Read the model definition and answer for the solid it produces. Units are mm, in the model's axes. A direction names the side the tool comes from. Give positions to 0.01 mm unless a question says otherwise; leave off trailing zeros. Order: outer loops, then holes, each group sorted by start corner. A loop starts at its lowest first (then second) coordinate and runs counter-clockwise, first axis right, second up.
Item 1: A cutting plane is placed at C-C (y = -8.5). Write down the section's boundary in (x, z).
Item 2: Which of the six approach directions +Z, -Z, +X, -X, +Y, -Y give full straight-line access (tool end or side, diameter ignored) to faces 1 (the face through (-9.19, -17.68, 3.45)), 2 (the face through (5.75, 6.62, 3.45))?
Item 3: Find the intervals of material crossed by line 1 along Y through (x, z) = (-3.75, 2.5); line 2 along Y through (x, z) = (-4.25, 5.5); line 3 along X through (y, z) = (-10, 3.75), in increasing order.
Item 4: The mould has two halves that part along X. Classify faces 3 (the face through (10.2, 0, 3)), 4 (the face through (5.8, -6.71, 3.45)), 5 (the face through (-9.19, 17.68, 3.45)), 6 (the face through (0, 18.668, 3)): +X half, -X half, draft (parallel to the pull), parting line (faces both ways), or undercut.
Item 5: A cutting plane is placed at B-B (z = 0.5). Write down the section's boundary in (x, y), plus the area to 3 significant figures.
Item 6: Given pin 1 Ø2 at (x, y) = (6, -1) entering from -Z, flat-ended and moving along its own axis, determine where the tip first touches the part or whether it passes through.
Item 7: A cutting plane is placed at D-D (x = 4.25). Write down the section's boundary in (y, z), plus the area to 3 significant figures.
Item 8: A cutting plane is placed at A-A (x = 1.5). Write down the section's boundary in (y, z), plus the area to 3 significant figures.
from build123d import *

# Parameters (mm, degrees)
SKETCH_W     = 20.4
SKETCH_H     = 37.336792
PAD_DEPTH    = 7
CHAMFER_SIZE = 2


with BuildPart() as part:
    # Sketch → Pad (new body)
    with BuildSketch(Plane.XY):
        Rectangle(SKETCH_W, SKETCH_H)
        Polygon((3.85, 16.668396), (-3.85, 16.668396), (-7.7, 10), (-3.85, 3.331604), (3.85, 3.331604), (7.7, 10), align=None, mode=Mode.SUBTRACT)
        Polygon((3.85, -3.331604), (-3.85, -3.331604), (-7.7, -10), (-3.85, -16.668396), (3.85, -16.668396), (7.7, -10), align=None, mode=Mode.SUBTRACT)
    extrude(amount=PAD_DEPTH)

    # Chamfer
    chamfer_edges = [part.edges().sort_by_distance(p)[0] for p in [
        (10.2, 18.668396, 3.5),
        (-10.2, 18.668396, 3.5),
        (10.2, -18.668396, 3.5),
        (-10.2, -18.668396, 3.5),
    ]]
    chamfer(chamfer_edges, length=CHAMFER_SIZE)


solid = part.part
Response values:
1. outline: (-10.2, 0) - (-6.83, 0) - (-6.83, 7) - (-10.2, 7) - close; (6.83, 0) - (10.2, 0) - (10.2, 7) - (6.83, 7) - close
2. face 1: +Z, -Z, -X, -Y
2. face 2: +Z, -Z
3. line 1: y = -18.67 to -16.67, -3.33 to 3.33, 16.67 to 18.67
3. line 2: y = -18.67 to -15.98, -4.02 to 4.02, 15.98 to 18.67
3. line 3: x = -10.2 to -7.7, 7.7 to 10.2
4. face 3: +X half
4. face 4: undercut
4. face 5: -X half
4. face 6: draft
5. outline: (-10.2, -16.67) - (-8.2, -18.67) - (8.2, -18.67) - (10.2, -16.67) - (10.2, 16.67) - (8.2, 18.67) - (-8.2, 18.67) - (-10.2, 16.67) - close; hole (-7.7, -10) - (-3.85, -16.67) - (3.85, -16.67) - (7.7, -10) - (3.85, -3.33) - (-3.85, -3.33) - close; hole (-7.7, 10) - (-3.85, 3.33) - (3.85, 3.33) - (7.7, 10) - (3.85, 16.67) - (-3.85, 16.67) - close
5. area: 446 mm2
6. pin 1: stops at z = 0
7. outline: (-18.67, 0) - (-15.98, 0) - (-15.98, 7) - (-18.67, 7) - close; (-4.02, 0) - (4.02, 0) - (4.02, 7) - (-4.02, 7) - close; (15.98, 0) - (18.67, 0) - (18.67, 7) - (15.98, 7) - close
7. area: 94.0 mm2
8. outline: (-18.67, 0) - (-16.67, 0) - (-16.67, 7) - (-18.67, 7) - close; (-3.33, 0) - (3.33, 0) - (3.33, 7) - (-3.33, 7) - close; (16.67, 0) - (18.67, 0) - (18.67, 7) - (16.67, 7) - close
8. area: 74.6 mm2
